Here's the drawing with two shaded views (mm, measured from the low corner). I have some questions. Give positions to 0.01 mm unless a question says otherwise; leave off trailing zeros. Loops run counter-clockwise (first coordinate to the right, second up) from the corner with the lowest first, then second, coordinate; pieces in that order, holes last. Notation, with made-up numbers: M -13.75,17 L 14.25,17 A17 cw 14.25,39 Z; hole C -2.5,21.5 d10. An arc over 180 degrees is marked long. Use CSV: the item, a comma, the result in double quotes.
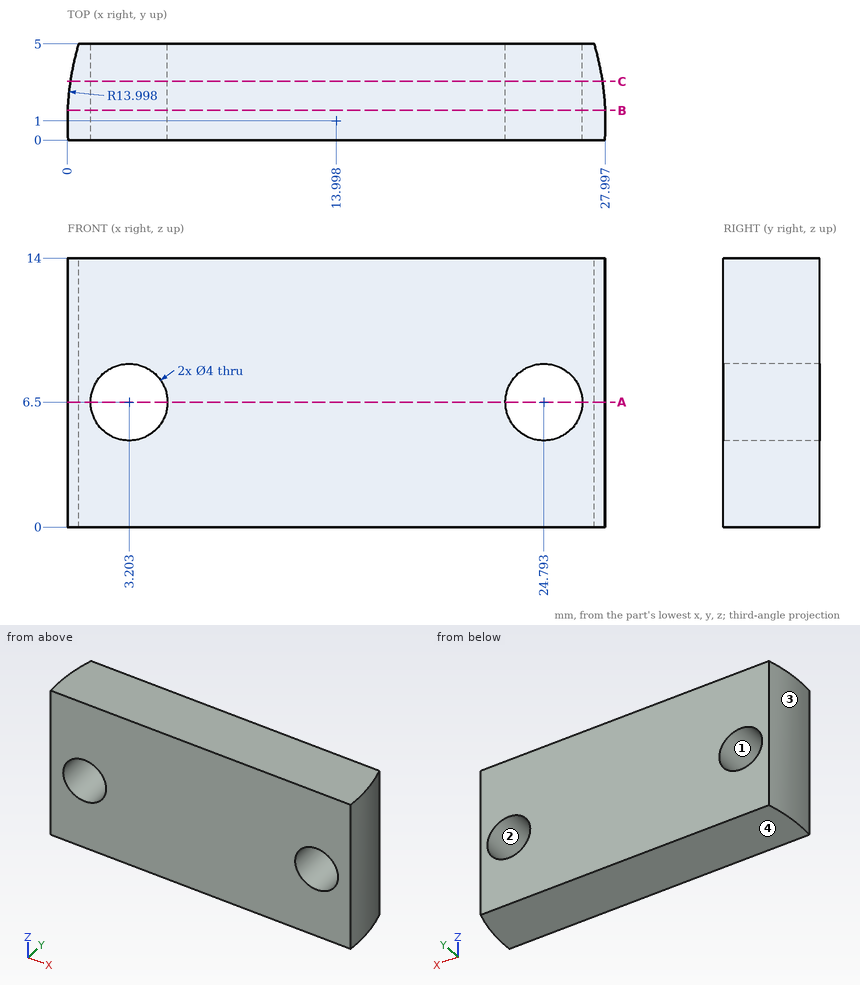
1. I want a section at A-A, the plane z = 6.5. List the corners of the cut face in (x, y) for me (1 decimal).
Outcome:
outline,"M 0,0 L 1.2,0 L 1.2,5 L 0.6,5 A14 ccw Z; M 5.2,0 L 22.8,0 L 22.8,5 L 5.2,5 Z; M 26.8,0 L 28,0 A14 ccw 27.4,5 L 26.8,5 Z"
2. If we mould it in two halves opening along X, with no side actions, what happens to the marked faces 1, 2, 3 and 4? For each: +X half, -X half, draft (parallel to the pull), parting line (faces both ways), or undercut.
Outcome:
face 1,"undercut"
face 2,"undercut"
face 3,"-X half"
face 4,"draft"
3. I want a section at B-B, the plane y = 1.55. List the corners of the cut face in (x, z) for me.
Outcome:
outline,"M 0.01,0 L 27.99,0 L 27.99,14 L 0.01,14 Z; hole C 3.2,6.5 d4; hole C 24.79,6.5 d4"
4. Please list where these lines run through material, in increasing order: line 1 (X direction, y = 4.6, z = 6.75) (1 decimal); line 2 (X direction, y = 3.3, z = 6.5); line 3 (X direction, y = 0.7, z = 3.25).
Outcome:
line 1,"0.5 to 1.2, 5.2 to 22.8, 26.8 to 27.5"
line 2,"0.19 to 1.2, 5.2 to 22.79, 26.79 to 27.81"
line 3,"0 to 27.99"
5. I want a section at C-C, the plane y = 3.05. List the corners of the cut face in (x, z) for me.
Outcome:
outline,"M 0.15,0 L 27.85,0 L 27.85,14 L 0.15,14 Z; hole C 3.2,6.5 d4; hole C 24.79,6.5 d4"
